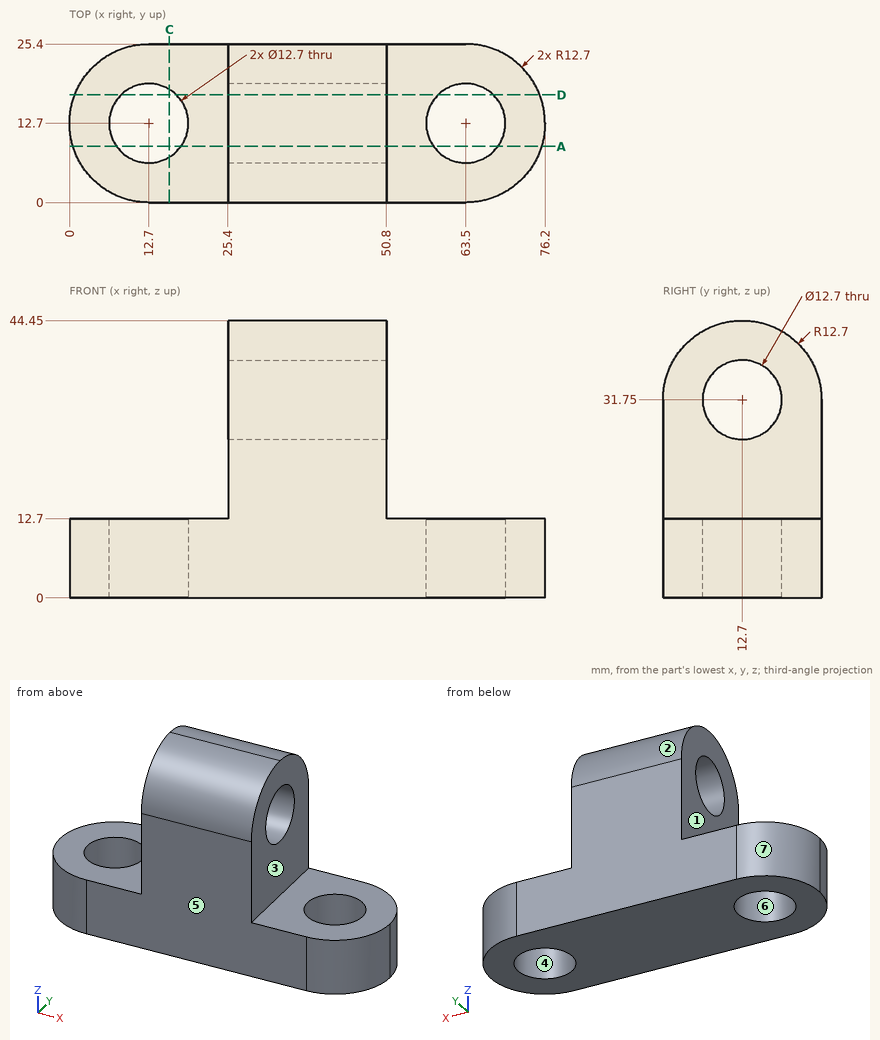
Answer from the drawing. Dimensions are ordinates in mm from the lowest x, y and z of the part. A direction names the side the tool comes from. Round coordinates to 2 decimals unless told otherwise and drop trailing zeros. Loops run counter-clockwise (first coordinate to the right, second up) from the corner with the lowest first, then second, coordinate; pieces in that order, holes last. Notation, with made-up numbers: (-29, 29.5) - (24, 29.5) arc R14 ccw to (24, 48.5) - close; hole circle Ø9 at (87.25, -29.5). An arc over 180 degrees is marked (long way). One line per item, written item: value.
Q1. Straight lines are drawn through the part: probe 1 along X at (y, z) = (17.75, 12.5); probe 2 along Z at (x, y) = (54, 4.25); probe 3 along X at (y, z) = (3.5, 19.5). For each, find the intervals that lie inside material, in ascending order.
Check values:
probe 1: 1.05 to 8.85, 16.55 to 59.65, 67.35 to 75.15
probe 2: 0 to 12.7
probe 3: 25.4 to 50.8
Q2. The mould has two halves that part along X. Classify the marked faces 4, 5, 6 and 7: +X half, -X half, draft (parallel to the pull), parting line (faces both ways), or undercut.
Check values:
face 4: undercut
face 5: draft
face 6: undercut
face 7: -X half
Q3. For the marked faces 1, 2 and 3, determine the directions among +Z, -Z, +X, -X, +Y, -Y from which every point of the face is accessible in a straight line to the end or side of a thin tool.
Check values:
face 1: +Z, -X, +Y, -Y
face 2: +Z, +X, -X, +Y
face 3: +Z, +X, +Y, -Y
Q4. Each of these flat-tipped pins is pushed along its axis until it touches: pin 1 Ø7.5 at (x, y) = (12.7, 12.7) entering from +Z; pin 2 Ø3 at (x, y) = (56, 10) entering from +Z; pin 3 Ø5 at (y, z) = (18, 10.5) entering from -X; pin 4 Ø1.5 at (x, y) = (36, 8.5) entering from +Z. Where does it stop, or does it pass through?
Check values:
pin 1: through
pin 2: z = 12.7
pin 3: x = 0.31
pin 4: z = 43.97
Q5. Find section D-D on y = 17.25. Give the vertices of the cut face in (x, z), and give its area (3 significant figures).
Check values:
outline: (0.84, 0) - (8.27, 0) - (8.27, 12.7) - (0.84, 12.7) - close; (17.13, 0) - (59.07, 0) - (59.07, 12.7) - (50.8, 12.7) - (50.8, 27.32) - (25.4, 27.32) - (25.4, 12.7) - (17.13, 12.7) - close; (25.4, 36.18) - (50.8, 36.18) - (50.8, 43.61) - (25.4, 43.61) - close; (67.93, 0) - (75.36, 0) - (75.36, 12.7) - (67.93, 12.7) - close
area: 1,280 mm2
Q6. Find section C-C on x = 16. Give the vertices of the cut face in (y, z).
Check values:
outline: (0, 0) - (7.27, 0) - (7.27, 12.7) - (0, 12.7) - close; (18.13, 0) - (25.4, 0) - (25.4, 12.7) - (18.13, 12.7) - close
Q7. Find section A-A on y = 9. Give the vertices of the cut face in (x, z), and give its area (3 significant figures).
Check values:
outline: (0.55, 0) - (7.54, 0) - (7.54, 12.7) - (0.55, 12.7) - close; (17.86, 0) - (58.34, 0) - (58.34, 12.7) - (50.8, 12.7) - (50.8, 26.59) - (25.4, 26.59) - (25.4, 12.7) - (17.86, 12.7) - close; (25.4, 36.91) - (50.8, 36.91) - (50.8, 43.9) - (25.4, 43.9) - close; (68.66, 0) - (75.65, 0) - (75.65, 12.7) - (68.66, 12.7) - close
area: 1,220 mm2
